Part model, mm, in its own coordinate system. A direction names the side the tool comes from. Coordinates: 2 decimals unless noted, no trailing zeros. Write item = value, one per line. Start each with the question number.
from build123d import *

# Parameters (mm, degrees)
SKETCH5_R               = 11
CUT_EXTRUDE1_DEPTH      = 7
SKETCH6_R               = 9.5
CUT_EXTRUDE2_DEPTH      = 8
CUT_EXTRUDE2_DEPTH_BACK = 28.879225258
CUT_EXTRUDE3_DEPTH      = 1
CUT_EXTRUDE3_DEPTH_BACK = 35.879225258


with BuildPart() as part:
    # Sketch2 → Revolve1 (revolve)
    with BuildSketch(Plane.XY):
        with BuildLine():
            Line((-14.019353848, 46.058143157), (14.019353848, 46.058143157))
            ThreePointArc((14.019353848, 46.058143157), (15.183914743, 48.1633599), (17.439612629, 49))
            Line((17.439612629, 49), (17.437695742, 49.258564993))
            ThreePointArc((17.437695742, 49.258564993), (-0.129286049, 66.439133401), (-17.439612629, 49))
            ThreePointArc((-17.439612629, 49), (-15.183914743, 48.1633599), (-14.019353848, 46.058143157))
        make_face()
    revolve(axis=Axis((-19.645151391, 0, 0), (1, 0, 0)))

    # Sketch4 → Revolve2 (revolve)
    with BuildSketch(Plane.XY):
        with BuildLine():
            Line((-14.019353848, 46.058143157), (14.019353848, 46.058143157))
            ThreePointArc((14.019353848, 46.058143157), (15.183914743, 48.1633599), (17.439612629, 49))
            Line((17.439612629, 49), (17.439612629, 0))
            Line((17.439612629, 0), (-17.439612629, 0))
            Line((-17.439612629, 0), (-17.439612629, 49))
            ThreePointArc((-17.439612629, 49), (-15.183914743, 48.1633599), (-14.019353848, 46.058143157))
        make_face()
    revolve(axis=Axis((-17.439612629, 0, 0), (1, 0, 0)))

    # Sketch5 → Cut-Extrude1 (cut)
    with BuildSketch(Plane(origin=(17.439612629, 0, 0), x_dir=(0, 0, -1), z_dir=(1, 0, 0))):
        Circle(SKETCH5_R)
    cut_extrude1 = extrude(amount=-CUT_EXTRUDE1_DEPTH, mode=Mode.SUBTRACT)

    # Mirror1: Cut-Extrude1 across plane
    add(cut_extrude1.mirror(Plane(origin=(0, 0, 0), x_dir=(0, 0, 1), z_dir=(1, 0, 0))), mode=Mode.SUBTRACT)

    # Sketch6 → Cut-Extrude2 (cut, two sides)
    with BuildSketch(Plane(origin=(10.439612629, 0, 0), x_dir=(0, 0, -1), z_dir=(1, 0, 0))) as cut_extrude2_sk:
        Circle(SKETCH6_R)
    extrude(amount=CUT_EXTRUDE2_DEPTH, mode=Mode.SUBTRACT)
    extrude(cut_extrude2_sk.sketch, amount=-CUT_EXTRUDE2_DEPTH_BACK, mode=Mode.SUBTRACT)

    # Sketch7 → Cut-Extrude3 (cut, two sides)
    with BuildSketch(Plane(origin=(17.439612629, 0, 0), x_dir=(0, 0, -1), z_dir=(1, 0, 0))) as cut_extrude3_sk:
        with BuildLine():
            Line((0.953103894, 14.00157653), (10.025977251, 42.574457114))
            ThreePointArc((10.025977251, 42.574457114), (9.781854194, 44.625759604), (8.07749124, 45.793057719))
            ThreePointArc((8.07749124, 45.793057719), (0, 46.5), (-8.07749124, 45.793057719))
            ThreePointArc((-8.07749124, 45.793057719), (-9.781854194, 44.625759604), (-10.025977251, 42.574457114))
            Line((-10.025977251, 42.574457114), (-0.953103894, 14.00157653))
            ThreePointArc((-0.953103894, 14.00157653), (0, 13.304219832), (0.953103894, 14.00157653))
        make_face()
        with BuildLine():
            Line((10.352622778, 9.475006807), (27.034956351, 34.383364488))
            ThreePointArc((27.034956351, 34.383364488), (28.790937454, 35.471467579), (30.766220791, 34.866741434))
            ThreePointArc((30.766220791, 34.866741434), (36.355163935, 28.992275786), (40.838687616, 22.236267533))
            ThreePointArc((40.838687616, 22.236267533), (40.988710121, 20.175944447), (39.53714549, 18.706115173))
            Line((39.53714549, 18.706115173), (11.541123893, 7.984673547))
            ThreePointArc((11.541123893, 7.984673547), (10.401657915, 8.295045387), (10.352622778, 9.475006807))
        make_face()
        with BuildLine():
            Line((13.862613343, -2.186436297), (43.738016408, 0.300897109))
            ThreePointArc((43.738016408, 0.300897109), (45.683565971, -0.393563019), (46.442341049, -2.314942302))
            ThreePointArc((46.442341049, -2.314942302), (45.334147916, -10.347223429), (42.84751926, -18.064885642))
            ThreePointArc((42.84751926, -18.064885642), (41.330231309, -19.466768393), (39.276036765, -19.248313029))
            Line((39.276036765, -19.248313029), (13.438442206, -4.044851475))
            ThreePointArc((13.438442206, -4.044851475), (12.970655264, -2.960467423), (13.862613343, -2.186436297))
        make_face()
        with BuildLine():
            Line((6.933773315, -12.201448274), (27.505458017, -34.00815193))
            ThreePointArc((27.505458017, -34.00815193), (28.175537537, -35.962232636), (27.146431247, -37.753427269))
            ThreePointArc((27.146431247, -37.753427269), (20.175593869, -41.895052357), (12.591294971, -44.762811473))
            ThreePointArc((12.591294971, -44.762811473), (10.549245338, -44.450607583), (9.43927127, -42.708368926))
            Line((9.43927127, -42.708368926), (5.216339443, -13.028520837))
            ThreePointArc((5.216339443, -13.028520837), (5.772484647, -11.986687881), (6.933773315, -12.201448274))
        make_face()
        with BuildLine():
            Line((-5.216339443, -13.028520837), (-9.43927127, -42.708368926))
            ThreePointArc((-9.43927127, -42.708368926), (-10.549245338, -44.450607583), (-12.591294971, -44.762811473))
            ThreePointArc((-12.591294971, -44.762811473), (-20.175593869, -41.895052357), (-27.146431247, -37.753427269))
            ThreePointArc((-27.146431247, -37.753427269), (-28.175537537, -35.962232636), (-27.505458017, -34.00815193))
            Line((-27.505458017, -34.00815193), (-6.933773315, -12.201448274))
            ThreePointArc((-6.933773315, -12.201448274), (-5.772484647, -11.986687881), (-5.216339443, -13.028520837))
        make_face()
        with BuildLine():
            Line((-13.438442206, -4.044851475), (-39.276036765, -19.248313029))
            ThreePointArc((-39.276036765, -19.248313029), (-41.330231309, -19.466768393), (-42.84751926, -18.064885642))
            ThreePointArc((-42.84751926, -18.064885642), (-45.334147916, -10.347223429), (-46.442341049, -2.314942302))
            ThreePointArc((-46.442341049, -2.314942302), (-45.683565971, -0.393563019), (-43.738016408, 0.300897109))
            Line((-43.738016408, 0.300897109), (-13.862613343, -2.186436297))
            ThreePointArc((-13.862613343, -2.186436297), (-12.970655264, -2.960467423), (-13.438442206, -4.044851475))
        make_face()
        with BuildLine():
            Line((-11.541123893, 7.984673547), (-39.53714549, 18.706115173))
            ThreePointArc((-39.53714549, 18.706115173), (-40.988710121, 20.175944447), (-40.838687616, 22.236267533))
            ThreePointArc((-40.838687616, 22.236267533), (-36.355163935, 28.992275786), (-30.766220791, 34.866741434))
            ThreePointArc((-30.766220791, 34.866741434), (-28.790937454, 35.471467579), (-27.034956351, 34.383364488))
            Line((-27.034956351, 34.383364488), (-10.352622778, 9.475006807))
            ThreePointArc((-10.352622778, 9.475006807), (-10.401657915, 8.295045387), (-11.541123893, 7.984673547))
        make_face()
        with BuildLine():
            Line((4.734554138, 14.392730444), (12.402770228, 38.541973357))
            ThreePointArc((12.402770228, 38.541973357), (20.175593869, 41.895052357), (22.400327415, 33.727403566))
            Line((22.400327415, 33.727403566), (8.300743558, 12.675344134))
            ThreePointArc((8.300743558, 12.675344134), (5.772484647, 11.986687881), (4.734554138, 14.392730444))
        make_face()
        with BuildLine():
            Line((14.204636001, 5.272097172), (37.866328919, 14.333651097))
            ThreePointArc((37.866328919, 14.333651097), (45.334147916, 10.347223429), (40.335521631, 3.515410976))
            Line((40.335521631, 3.515410976), (15.085412051, 1.413165161))
            ThreePointArc((15.085412051, 1.413165161), (12.970655264, 2.960467423), (14.204636001, 5.272097172))
        make_face()
        with BuildLine():
            Line((12.978337234, -7.818532802), (34.815769602, -20.668202792))
            ThreePointArc((34.815769602, -20.668202792), (36.355163935, -28.992275786), (27.897245365, -29.34375778))
            Line((27.897245365, -29.34375778), (10.510457583, -10.913156002))
            ThreePointArc((10.510457583, -10.913156002), (10.401657915, -8.295045387), (12.978337234, -7.818532802))
        make_face()
        with BuildLine():
            Line((1.979085819, -15.021648107), (5.548225662, -40.106478424))
            ThreePointArc((5.548225662, -40.106478424), (0, -46.5), (-5.548225662, -40.106478424))
            Line((-5.548225662, -40.106478424), (-1.979085819, -15.021648107))
            ThreePointArc((-1.979085819, -15.021648107), (0, -13.304219832), (1.979085819, -15.021648107))
        make_face()
        with BuildLine():
            Line((-10.510457583, -10.913156002), (-27.897245365, -29.34375778))
            ThreePointArc((-27.897245365, -29.34375778), (-36.355163935, -28.992275786), (-34.815769602, -20.668202792))
            Line((-34.815769602, -20.668202792), (-12.978337234, -7.818532802))
            ThreePointArc((-12.978337234, -7.818532802), (-10.401657915, -8.295045387), (-10.510457583, -10.913156002))
        make_face()
        with BuildLine():
            Line((-15.085412051, 1.413165161), (-40.335521631, 3.515410976))
            ThreePointArc((-40.335521631, 3.515410976), (-45.334147916, 10.347223429), (-37.866328919, 14.333651097))
            Line((-37.866328919, 14.333651097), (-14.204636001, 5.272097172))
            ThreePointArc((-14.204636001, 5.272097172), (-12.970655264, 2.960467423), (-15.085412051, 1.413165161))
        make_face()
        with BuildLine():
            Line((-8.300743558, 12.675344134), (-22.400327415, 33.727403566))
            ThreePointArc((-22.400327415, 33.727403566), (-20.175593869, 41.895052357), (-12.402770228, 38.541973357))
            Line((-12.402770228, 38.541973357), (-4.734554138, 14.392730444))
            ThreePointArc((-4.734554138, 14.392730444), (-5.772484647, 11.986687881), (-8.300743558, 12.675344134))
        make_face()
    extrude(amount=CUT_EXTRUDE3_DEPTH, mode=Mode.SUBTRACT)
    extrude(cut_extrude3_sk.sketch, amount=-CUT_EXTRUDE3_DEPTH_BACK, mode=Mode.SUBTRACT)


solid = part.part
Item 1: 3-axis set-ups, long thin cutter, end or side, ignore diameter. For faces 3 (the flat face through (17.44, 11, 4)), 4 (the cylindrical face through (0.244, -41.944, 20.073)): which of +Z, -Z, +X, -X, +Y, -Y reach the whole face in a straight line?
Item 2: Wall check: line 1 along Y through (x, z) = (11.5, 26); line 2 along Y through (x, z) = (9.5, -40.5); line 3 along Z through (x, y) = (7, -26.5). Give the ranges that are in metal, low to high. Write a range as [from, to].
Item 3: Cut at A-A, the plane x = -7. Count the separate pieces of the cut face and the enclosed holes in it, and give its area (3 significant figures).
Item 4: Flat gauge pins, fed straight in: pin 1 (2 mm diameter, centred on x = 5.5, z = 22, fed in from -Y); pin 2 (1 mm diameter, centred on x = -0.5, z = 3.5, fed in from +Y); pin 3 (6 mm diameter, centred on x = -12, z = -33.5, fed in from -Y). Where does each tip first touch, or does it go through?
Item 5: Pull direction Y, two halves, no side cores. Call faces 1 (the flat face through (-17.44, 11, -3)), 2 (the flat face through (0.24, 23.05, 15.25)): pulls with the +Y half, pulls with the -Y half, needs draft (parallel to the pull), parting line crosses it, or undercut.
Filled sheet:
q1.face_3 = +Z, -Z, +X, +Y, -Y
q1.face_4 = +X, -X
q2.line_1 = [-56.41, -38.55], [-32.41, -27.33], [-15.48, -11.44], [-1.18, 2.32], [9.79, 13.52], [32.84, 56.41]
q2.line_2 = [-49.07, -19.59], [0.03, 3.53], [14.67, 19.37], [22.85, 49.07]
q2.line_3 = [-59.32, -37.49], [-25.21, -20.42], [-7.13, -3.61], [3.61, 7.13], [20.42, 25.21], [37.49, 59.32]
q3.separate_pieces = 1
q3.enclosed_holes = 15
q3.area = 8,520 mm2
q4.pin_1 = -62.23
q4.pin_2 = 66.37
q4.pin_3 = -55.09
q5.face_1 = needs draft
q5.face_2 = undercut
